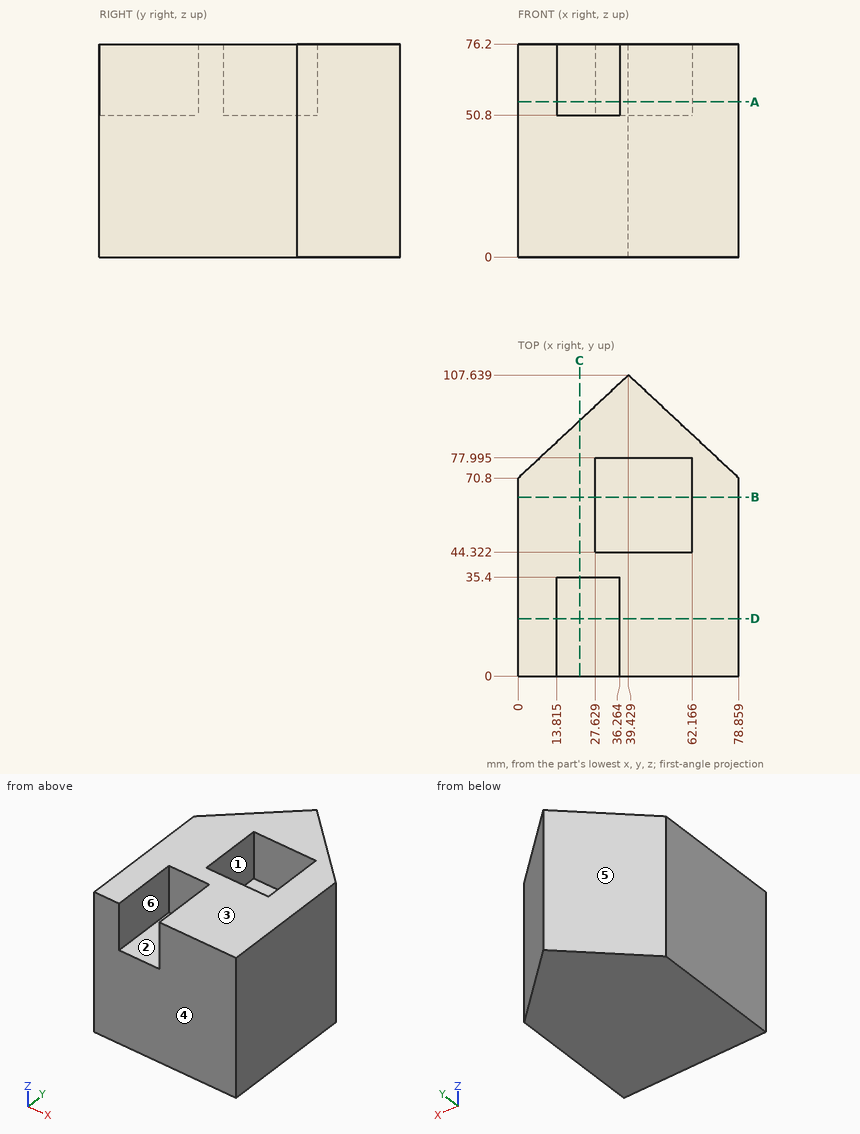
Part print with two shaded views. Sizes in mm from the minimum x, y, z corner. A direction names the side the tool comes from. Coordinates: 2 decimals unless noted, no trailing zeros. Loops run counter-clockwise (first coordinate to the right, second up) from the corner with the lowest first, then second, coordinate; pieces in that order, holes last. Notation, with made-up numbers: M 80.25,-30.5 L 99.25,-30.5 A17 ccw 99.25,-11.5 Z; hole C -7,66 d1. An arc over 180 degrees is marked long. Use CSV: the item, a comma, the result in double quotes. Start each with the question number.
1. Band-saw the part on C-C, the plane x = 22. List the corners of the cut face in (y, z) (1 decimal), then the cut area to 3 significant figures.
2. Band-saw the part on D-D, the plane y = 20.5. List the corners of the cut face in (x, z) (1 decimal), then the cut area to 3 significant figures.
3. Band-saw the part on B-B, the plane y = 64. List the corners of the cut face in (x, z), then the cut area to 3 significant figures.
4. Band-saw the part on A-A, the plane z = 55.5. List the corners of the cut face in (x, y) (1 decimal).
5. Two-plate mould, pull along X, no slides. Class the marked faces 4, 5 and 6: pulls with the +X half, pulls with the -X half, needs draft (parallel to the pull), parting line crosses it, or undercut.
6. Tool access for the marked faces 1, 2 and 3: list every direction of +Z, -Z, +X, -X, +Y, -Y with a clear straight run to the whole face (end or side of a thin tool).
7. Probe probe 1 along X at (y, z) = (24, 62) (1 decimal); probe 2 along Z at (x, y) = (17.5, 24); probe 3 along Y at (x, z) = (46, 67.5) (1 decimal). List the from-to ranges inside material, lowest first. Write a range as [from, to].
8. Flat gauge pins, fed straight in: pin 1 (4 mm diameter, centred on y = 80.5, z = 13.5, fed in from -X); pin 2 (12.5 mm diameter, centred on x = 47.5, z = 62.5, fed in from +Y); pin 3 (8 mm diameter, centred on x = 9, z = 24.5, fed in from +Y) (1 decimal). Where does each tip first touch, or does it go through?
Entries:
1,outline,"M 0,0 L 91.4,0 L 91.4,76.2 L 35.4,76.2 L 35.4,50.8 L 0,50.8 Z"
1,area,"6,060 mm2"
2,outline,"M 0,0 L 78.9,0 L 78.9,76.2 L 36.3,76.2 L 36.3,50.8 L 13.8,50.8 L 13.8,76.2 L 0,76.2 Z"
2,area,"5,440 mm2"
3,outline,"M 0,0 L 78.86,0 L 78.86,76.2 L 62.17,76.2 L 62.17,50.8 L 27.63,50.8 L 27.63,76.2 L 0,76.2 Z"
3,area,"5,130 mm2"
4,outline,"M 0,0 L 13.8,0 L 13.8,35.4 L 36.3,35.4 L 36.3,0 L 78.9,0 L 78.9,70.8 L 39.4,107.6 L 0,70.8 Z; hole M 27.6,44.3 L 62.2,44.3 L 62.2,78 L 27.6,78 Z"
5,face 4,"needs draft"
5,face 5,"pulls with the -X half"
5,face 6,"undercut"
6,face 1,"+Z"
6,face 2,"+Z, -Y"
6,face 3,"+Z, +X, -X, +Y, -Y"
7,probe 1,"x = [0, 13.8], [36.3, 78.9]"
7,probe 2,"z = [0, 50.8]"
7,probe 3,"y = [0, 44.3], [78, 101.5]"
8,pin 1,"stops at x = 8.24"
8,pin 2,"stops at y = 105.94"
8,pin 3,"stops at y = 82.9"
